Verification items for the finished model (mm, model axes). A direction names the side the tool comes from. Round coordinates to 2 decimals unless told otherwise and drop trailing zeros. Write each loop counter-clockwise with the first axis right and the second up, starting at its lowest first coordinate (ties: lowest second). Pieces come first, ordered by that corner, then holes. Notation, with made-up numbers: M -3.75,1.5 L 47.25,1.5 A22 cw 47.25,24.5 Z; hole C 22,-32.5 d10. An arc over 180 degrees is marked long. Use a Markdown table: item, result. Add a question column.
from build123d import *

# Parameters (mm, degrees)
SKETCH1_R           = 7.2
BOSS_EXTRUDE1_DEPTH = 2.95
SKETCH2_R           = 1.25
CUT_EXTRUDE1_DEPTH  = 5


with BuildPart() as part:
    # Sketch1 → Boss-Extrude1 (new, symmetric)
    with BuildSketch(Plane.XY):
        with BuildLine():
            Line((-9.992822271, 13.378817988), (-10.5, 0))
            Line((-10.5, 0), (10.5, 0))
            Line((10.5, 0), (9.992822271, 13.378817988))
            ThreePointArc((9.992822271, 13.378817988), (0, 23), (-9.992822271, 13.378817988))
        make_face()
        with Locations((0, 13)):
            Circle(SKETCH1_R, mode=Mode.SUBTRACT)
    extrude(amount=BOSS_EXTRUDE1_DEPTH, both=True)

    # Sketch2 → Cut-Extrude1 (cut)
    with BuildSketch(Plane.XZ):
        with Locations(Location((-6.95, 0, 0), (0, 0, 270))):
            Circle(SKETCH2_R)
        with Locations(Location((6.95, 0, 0), (0, 0, 270))):
            Circle(SKETCH2_R)
    extrude(amount=-CUT_EXTRUDE1_DEPTH, mode=Mode.SUBTRACT)


solid = part.part
1. Cross-section at C-C on y = 10.25. Enter the section's corners in (x, z).
2. Depth check by flat-ended pin: pin 1 Ø2 at (y, z) = (20.5, -0.5) entering from +X; pin 2 Ø1.5 at (x, z) = (-1, 2) entering from +Y; pin 3 Ø3 at (x, z) = (6.95, 0) entering from +Y. Enter the tip coordinate at first touch or a pass-through.
3. Access from +Z, -Z, +X, -X, +Y, -Y to the whole of each face (thin tool, end or side, straight path). Record for faces 4 (the flat face through (7, 5, 0)), 5 (the flat face through (0, 0, 0)).
4. Release check for a two-part mould opening along Z. For faces 1 (the flat face through (-7, 5, 0)), 2 (the flat face through (-10.243, 6.783, 0.041)), 3 (the flat face through (0, 4, 2.95)) record: +Z half, -Z half, draft (parallel to the pull), parting line (faces both ways), or undercut.
5. Cross-section at B-B on z = 0. Enter the section's corners in (x, y).
6. Cross-section at A-A on x = 0. Enter the section's corners in (y, z).
7. Cross-section at D-D on z = -2.05. Enter the section's corners in (x, y), plus the area to 3 significant figures.
8. Scan lines: line 1 along X through (y, z) = (1.7, 0); line 2 along Y through (x, z) = (0, -0.7); line 3 along X through (y, z) = (4, 0). Record each from-to range of solid material in increasing order. Write a range as from..to.
Answer:
| question | item | result |
|---|---|---|
| 1 | outline | M -10.11,-2.95 L -6.65,-2.95 L -6.65,2.95 L -10.11,2.95 Z; M 6.65,-2.95 L 10.11,-2.95 L 10.11,2.95 L 6.65,2.95 Z |
| 2 | pin 1 | stops at x = 7.6 |
| 2 | pin 2 | stops at y = 23 |
| 2 | pin 3 | stops at y = 21.38 |
| 3 | face 4 | -Y |
| 3 | face 5 | +Z, -Z, +X, -X, -Y |
| 4 | face 1 | undercut |
| 4 | face 2 | draft |
| 4 | face 3 | +Z half |
| 5 | outline | M -10.5,0 L -8.2,0 L -8.2,5 L -5.7,5 L -5.7,0 L 5.7,0 L 5.7,5 L 8.2,5 L 8.2,0 L 10.5,0 L 9.99,13.38 A10 ccw -9.99,13.38 Z; hole C 0,13 d14.4 |
| 6 | outline | M 0,-2.95 L 5.8,-2.95 L 5.8,2.95 L 0,2.95 Z; M 20.2,-2.95 L 23,-2.95 L 23,2.95 L 20.2,2.95 Z |
| 7 | outline | M -10.5,0 L 10.5,0 L 9.99,13.38 A10 ccw -9.99,13.38 Z; hole C 0,13 d14.4 |
| 7 | area | 261 mm^2 |
| 8 | line 1 | x = -10.44..-8.2, -5.7..5.7, 8.2..10.44 |
| 8 | line 2 | y = 0..5.8, 20.2..23 |
| 8 | line 3 | x = -10.35..-8.2, -5.7..5.7, 8.2..10.35 |
